The model under review builds one solid part; all positions refer to its coordinate system, in mm. A direction names the side the tool comes from. Give positions to 0.01 mm unless a question says otherwise; leave off trailing zeros. Loops run counter-clockwise (first coordinate to the right, second up) from the corner with the lowest first, then second, coordinate; pieces in that order, holes last. Notation, with made-up numbers: M 45.25,-7 L 78.25,-7 A21 cw 78.25,8 Z; hole C 2,59.5 d2. An arc over 180 degrees is marked long. One line per item, written item: value. Start each with the question number.
Q1. We need section B-B on z = -31. Write out the cut boundary in (x, y).
Q2. For faces 4 (the face through (10.537, 2.021, 49.248)), 5 (the face through (6.3, 2, -31)), 6 (the face through (-0.1, 1.1, 15.6)), list the 3-axis set-ups (+Z, -Z, +X, -X, +Y, -Y) from which the entire face can be reached by the end or side of a thin tool; tool diameter is ignored.
Q3. To check wall thickness, follow line 1 along Z through (x, y) = (-2.75, 0.75); line 2 along Z through (x, y) = (-3, 2.6); line 3 along Z through (x, y) = (0, 3.9) (3 decimals). State the ranges of each line that lie inside material, in increasing order. Write a range as from..to.
Q4. Mouldability with a two-part tool opening along Z and no side actions: class faces 1 (the face through (0, 1, -47.35)), 2 (the face through (0, 4.1, 1)), 3 (the face through (-10.498, 2.021, 49.287)) as released by +Z, released by -Z, zero draft, split by the parting line, or undercut.
Q5. We need section A-A on x = -2.5. Write out the cut boundary in (y, z), plus the area to 3 significant figures.
Q6. For pin 1 (2.5 mm diameter, centred on x = 2.5, z = 46, fed in from +Y); pin 2 (5 mm diameter, centred on x = 0, z = -44.925, fed in from -Y); pin 3 (4 mm diameter, centred on x = -3, z = -18, fed in from -Y), all flat-tipped, find the tip position at first contact; note any pin that passes through.
Autodesk Inventor part; units mm, degrees
ref_plane "YZ Plane" through (0, 0, 0) normal (1, 0, 0) x (0, 1, 0)
ref_plane "XZ Plane" through (0, 0, 0) normal (0, 1, 0) x (-1, 0, 0)
ref_plane "XY Plane" through (0, 0, 0) normal (0, 0, 1) x (1, 0, 0)
sketch "Szkic1" plane through (0, 0, 0) normal (0, 1, 0) x (-1, 0, 0)
  line L0 (8.75, 50) -> (-8.75, 50)
  line L1 (-11.25, 47.5) -> (-11.25, -47.5)
  line L2 (-8.75, -50) -> (8.75, -50)
  line L3 (11.25, -47.5) -> (11.25, 47.5)
  line L4 (-11.25, 50) -> (11.25, -50)
  line L5 (-11.25, -50) -> (11.25, 50)
  arc A0 (11.25, 47.5) -> (8.75, 50) centre (8.75, 47.5) ccw
  arc A1 (-8.75, 50) -> (-11.25, 47.5) centre (-8.75, 47.5) ccw
  arc A2 (-11.25, -47.5) -> (-8.75, -50) centre (-8.75, -47.5) ccw
  arc A3 (8.75, -50) -> (11.25, -47.5) centre (8.75, -47.5) ccw
  point P0 (0, 0)
  point P1 (0, 0)
  dimension "d0" = 22.5
  dimension "d1" = 100
  dimension "d2" = 2.5
extrude "Wyciągnięcie proste1" add sketch "Szkic1" along normal blind 4.1
sketch "Szkic2" plane through (0, 4.1, 0) normal (0, 1, 0) x (1, 0, 0)
  line L0 (-6.3, -42.5) -> (6.3, -42.5)
  line L1 (6.3, -42.5) -> (6.3, -19.7)
  line L2 (6.3, -19.7) -> (-6.3, -19.7)
  line L3 (-6.3, -19.7) -> (-6.3, -42.5)
  line L4 (-8.75, -50) -> (8.75, -50)
  line L5 (11.25, -47.5) -> (11.25, 47.5)
  line L6 (-6.3, 19.7) -> (6.3, 19.7)
  line L7 (6.3, 19.7) -> (6.3, 42.5)
  line L8 (6.3, 42.5) -> (-6.3, 42.5)
  line L9 (-6.3, 42.5) -> (-6.3, 19.7)
  line L10 (-15.75, 0) -> (15.75, 0)
  point P0 (0, 0)
  point P1 (0, -42.5)
  dimension "d5" = 12.6
  dimension "d6" = 22.8
  dimension "d7" = 7.5
  dimension "d8" = 11.25
extrude "Wyciągnięcie proste2" cut sketch "Szkic2" against normal blind 4.1
sketch "Szkic4" plane through (0, 4.1, 0) normal (0, 1, 0) x (1, 0, 0)
  line L0 (-6.3, -47.35) -> (6.3, -47.35)
  line L1 (6.3, -47.35) -> (6.3, -14.85)
  line L2 (6.3, -14.85) -> (-6.3, -14.85)
  line L3 (-6.3, -14.85) -> (-6.3, -47.35)
  line L4 (6.3, -42.5) -> (-6.3, -42.5)
  line L5 (-6.3, -19.7) -> (6.3, -19.7)
  point P0 (0, 0)
  dimension "d11" = 4.85
  dimension "d12" = 4.85
extrude "Wyciągnięcie proste3" cut sketch "Szkic4" against normal blind 3 contours L3 L4 L1 L0 | L3 L2 L1 L5
sketch "Szkic5" plane through (0, 1.1, 0) normal (0, 1, 0) x (1, 0, 0)
  circle A0 centre (0, -44.925) radius 1.5
  circle A1 centre (0, -17.275) radius 1.5
  circle A2 centre (0, 17.275) radius 1.5
  circle A3 centre (0, 44.925) radius 1.5
  line L0 (-6.3, -42.5) -> (6.3, -42.5)
  line L1 (6.3, -19.7) -> (-6.3, -19.7)
  line L2 (-6.3, 19.7) -> (6.3, 19.7)
  line L3 (6.3, 42.5) -> (-6.3, 42.5)
  point P0 (0, 0)
  point P1 (0, -42.5)
  point P2 (0, -19.7)
  point P3 (0, 19.7)
  point P4 (0, 42.5)
  dimension "d17" = 3
  dimension "d18" = 3
  dimension "d19" = 3
  dimension "d20" = 3
  dimension "d21" = 2.425
  dimension "d22" = 2.425
  dimension "d23" = 2.425
  dimension "d24" = 2.425
extrude "Wyciągnięcie proste4" cut sketch "Szkic5" against normal blind 3
sketch "Szkic6" plane through (0, 0, 0) normal (0, -1, 0) x (1, 0, 0)
  line L0 (-6.3, -19.7) -> (6.3, -19.7)
  line L1 (6.3, -19.7) -> (6.3, -14.85)
  line L2 (6.3, -14.85) -> (-6.3, -14.85)
  line L3 (-6.3, -14.85) -> (-6.3, -19.7)
  line L4 (-6.3, -47.35) -> (6.3, -47.35)
  line L5 (6.3, -47.35) -> (6.3, -42.5)
  line L6 (6.3, -42.5) -> (-6.3, -42.5)
  line L7 (-6.3, -42.5) -> (-6.3, -47.35)
  point P0 (0, 0)
  dimension "d27" = 4.85
  dimension "d28" = 4.85
extrude "Wyciągnięcie proste5" cut sketch "Szkic6" against normal blind 3
sketch "Szkic7" plane through (0, 3, 0) normal (0, -1, 0) x (1, 0, 0)
  circle A0 centre (0, -44.925) radius 1.5
  circle A1 centre (0, -17.275) radius 1.5
  line L0 (6.3, -19.7) -> (-6.3, -19.7)
  line L1 (-6.3, -42.5) -> (6.3, -42.5)
  point P0 (0, 0)
  point P1 (0, -19.7)
  dimension "d31" = 3
  dimension "d32" = 3
  dimension "d33" = 2.425
  dimension "d34" = 2.425
extrude "Wyciągnięcie proste6" cut sketch "Szkic7" against normal blind 3
properties part number "arm_medium_part"
Solved:
1. outline: M -11.25,0 L -6.3,0 L -6.3,4.1 L -11.25,4.1 Z; M 6.3,0 L 11.25,0 L 11.25,4.1 L 6.3,4.1 Z
2. face 4: +Z, +X, +Y, -Y
2. face 5: -Y
2. face 6: +Y
3. line 1: -50..-47.35, -14.85..19.7, 42.5..50
3. line 2: -50..-47.35, -14.85..14.85, 47.35..50
3. line 3: -50..-46.425, -43.425..-42.5, -19.7..-18.775, -15.775..14.85, 47.35..50
4. face 1: undercut
4. face 2: zero draft
4. face 3: released by +Z
5. outline: M 0,-50 L 4.1,-50 L 4.1,-42.5 L 3,-42.5 L 3,-47.35 L 0,-47.35 Z; M 0,-14.85 L 3,-14.85 L 3,-19.7 L 4.1,-19.7 L 4.1,14.85 L 1.1,14.85 L 1.1,19.7 L 0,19.7 Z; M 0,42.5 L 1.1,42.5 L 1.1,47.35 L 4.1,47.35 L 4.1,50 L 0,50 Z
5. area: 165 mm2
6. pin 1: y = 1.1
6. pin 2: y = 0
6. pin 3: y = 3
